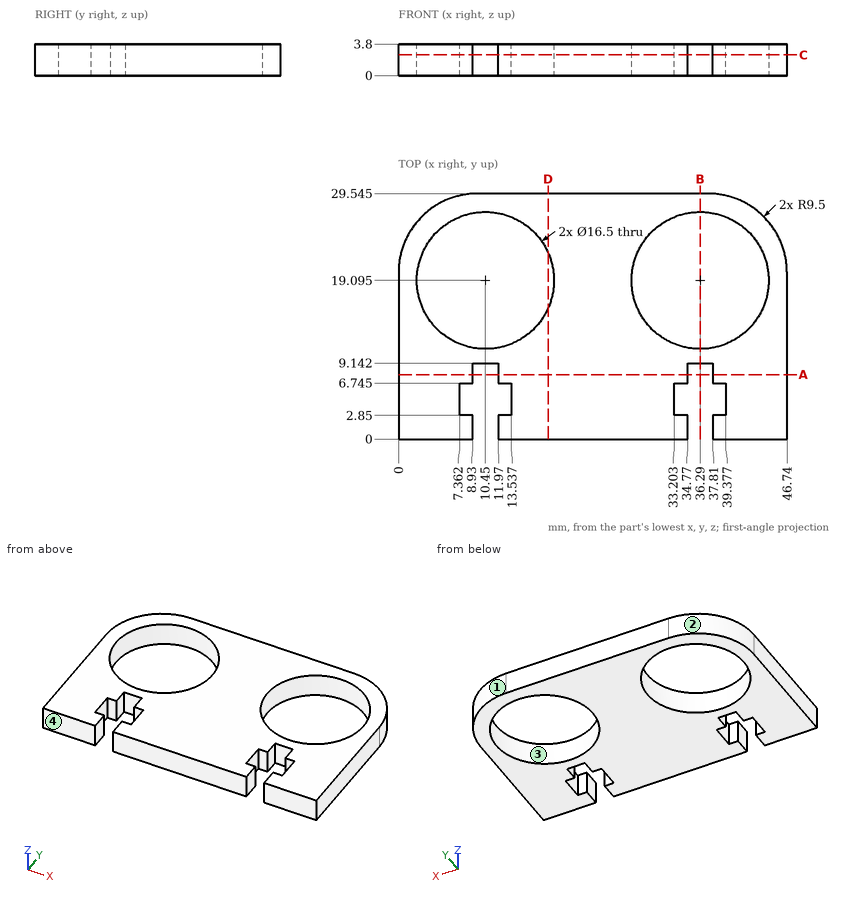
Here's the drawing with two shaded views (mm, measured from the low corner). I have some questions. Round coordinates to 2 decimals unless told otherwise and drop trailing zeros. Loops run counter-clockwise (first coordinate to the right, second up) from the corner with the lowest first, then second, coordinate; pieces in that order, holes last. Notation, with made-up numbers: M 46.25,-20.5 L 60.25,-20.5 A20 cw 60.25,-6.5 Z; hole C -26,62 d4. An arc over 180 degrees is marked long. Answer as a JSON object with one key per item and string values. Group by question number.
Q1. Imagine slicing it at A-A, the plane y = 7.75. Please give me the cut outline in (x, z).
Q2. Imagine slicing it at C-C, the plane z = 2.5. Count the separate pieces of the cut face and the enclosed holes in it.
Q3. Imagine slicing it at D-D, the plane x = 18. Please give me the cut outline in (y, z) (1 decimal).
Q4. Please list where these lines run through material, in increasing order: L1, parallel to X at y = 8, z = 3.65; L2, parallel to Y at x = 36.5, z = 0.3 (1 decimal); L3, parallel to X at y = 17.25, z = 3.3.
Q5. Imagine slicing it at B-B, the plane x = 36.29. Please give me the cut outline in (y, z) (1 decimal).
Q6. We'd pull the mould along X, two halves only. Please class the marked faces 1, 2, 3 and 4: +X half, -X half, draft (parallel to the pull), parting line (faces both ways), or undercut.
Q7. Will this pin go through, and if not, where does the flat tip stop? pin 1 (1 mm diameter, centred on x = 8, z = 2, fed in from +Y).
Findings:
{
 "1": {"outline": "M 0,0 L 8.93,0 L 8.93,3.8 L 0,3.8 Z; M 11.97,0 L 34.77,0 L 34.77,3.8 L 11.97,3.8 Z; M 37.81,0 L 46.74,0 L 46.74,3.8 L 37.81,3.8 Z"},
 "2": {"separate pieces": "1", "enclosed holes": "2"},
 "3": {"outline": "M 0,0 L 15.8,0 L 15.8,3.8 L 0,3.8 Z; M 22.4,0 L 29.5,0 L 29.5,3.8 L 22.4,3.8 Z"},
 "4": {"L1": "x = 0 to 8.93, 11.97 to 34.77, 37.81 to 46.74", "L2": "y = 9.1 to 10.8, 27.3 to 29.5", "L3": "x = 0 to 2.41, 18.49 to 28.25, 44.33 to 46.74"},
 "5": {"outline": "M 9.1,0 L 10.8,0 L 10.8,3.8 L 9.1,3.8 Z; M 27.3,0 L 29.5,0 L 29.5,3.8 L 27.3,3.8 Z"},
 "6": {"face 1": "+X half", "face 2": "-X half", "face 3": "undercut", "face 4": "draft"},
 "7": {"pin 1": "stops at y = 29.49"}
}
